Input: part model. Units: mm. Frame: model coordinates. A direction names the side the tool comes from. Coordinates: 2 decimals unless noted, no trailing zeros. Order: outer loops, then holes, each group sorted by start corner. A loop starts at its lowest first (then second) coordinate and runs counter-clockwise, first axis right, second up. Notation, with made-up numbers: (-14, 71.5) -> (4, 71.5) arc R14 cw to (4, 85.5) -> close; hole circle Ø7 at (53.5, 77). An arc over 180 degrees is marked (long way). Use one line per item in the form item = value. Start each with the question number.
1) Section query A-A on x = 24. Output: boundary loops of the cut face in (y, z).
2) Pin query (flat end, axial travel): pin 1 (1 mm diameter, centred on y = -1, z = -38, fed in from -X); pin 2 (10 mm diameter, centred on x = -24, z = -41, fed in from -Y); pin 3 (2 mm diameter, centred on x = 9.5, z = -51.5, fed in from +Y). Return the tip coordinate at first contact, or that it passes through.
3) Draft query along X for faces 1 (the cylindrical face through (43.998, 0.325, -57.664)), 2 (the cylindrical face through (-5.9, -44.934, -29.58)), 3 (the cylindrical face through (0.9, 44, -55)). Return one class per face: pulls with the +X half, pulls with the -X half, needs draft (parallel to the pull), parting line crosses it, or undercut.
4) Section query D-D on y = -6.5. Output: boundary loops of the cut face in (x, z).
5) Section query B-B on y = 12. Output: boundary loops of the cut face in (x, z), then the cut area to 3 significant figures.
6) Section query C-C on z = -35.2. Output: boundary loops of the cut face in (x, y) (3 decimals).
7) Ray query, line 1 along Z through (x, y) = (0, 43.95); line 2 along Z through (x, y) = (0, -43.8); line 3 along Y through (x, z) = (0, -28.5) (3 decimals). Return the intervals inside material, ascending.
8) Access query for faces 4 (the flat face through (44, 1.5, -9)), 5 (the cylindrical face through (40.7, -12.8, -29.6)), 6 (the flat face through (1.5, 44, -9)). Directions: +Z, -Z, +X, -X, +Y, -Y. A direction counts if a zero-diameter tool reaches every point of the face in a straight line with its end or side. Return the directions, or none.
from build123d import *

# Parameters (mm, degrees)
SKETCH_R             = 45.32
SKETCH_R_2           = 42.665
PAD_DEPTH            = 60
SKETCH002_R          = 1.5
SKETCH002_R_2        = 10
POCKET_DEPTH         = 8
SKETCH003_R          = 1.5
POCKET001_DEPTH      = 8
SKETCH004_R          = 1.5
POCKET002_DEPTH      = 5
BODY_PLACEMENT_ANGLE = 180


with BuildPart() as part:
    # Sketch → Pad (new body)
    with BuildSketch(Plane.XY):
        Circle(SKETCH_R)
        Circle(SKETCH_R_2, mode=Mode.SUBTRACT)
    extrude(amount=PAD_DEPTH)

    # Sketch002 (on DatumPlane) → Pocket (cut)
    with BuildSketch(Plane(origin=(45.32, 0, 60), x_dir=(0, 1, 0), z_dir=(-1, 0, 0))):
        with Locations((0, 3.8)):
            Circle(SKETCH002_R)
        with Locations((0, 18)):
            Circle(SKETCH002_R_2)
        with BuildLine():
            Line((0, 47.6), (0.0005, 47.6))
            ThreePointArc((0.0005, 47.6), (1.060807, 48.039193), (1.5, 49.0995))
            Line((1.5, 49.0995), (1.5, 52.1005))
            ThreePointArc((1.5, 52.1005), (1.060807, 53.160807), (0.0005, 53.6))
            Line((0.0005, 53.6), (0, 53.6))
            ThreePointArc((0, 53.6), (-1.06066, 53.16066), (-1.5, 52.1))
            Line((-1.5, 52.1), (-1.5, 49.1))
            ThreePointArc((-1.5, 49.1), (-1.06066, 48.03934), (0, 47.6))
        make_face()
    extrude(amount=POCKET_DEPTH, mode=Mode.SUBTRACT)

    # Sketch003 (on DatumPlane) → Pocket001 (cut)
    with BuildSketch(Plane(origin=(0, 45.32, 60), x_dir=(0, 0, -1), z_dir=(0, 1, 0))):
        with Locations((3.8, 0)):
            Circle(SKETCH003_R)
        with Locations((24.8, 0)):
            Circle(SKETCH003_R)
    extrude(amount=-POCKET001_DEPTH, mode=Mode.SUBTRACT)

    # Sketch004 (on DatumPlane) → Pocket002 (cut)
    with BuildSketch(Plane(origin=(0, -45.32, 60), x_dir=(0, 0, 1), z_dir=(0, -1, 0))):
        with Locations((-3.8, 0)):
            Circle(SKETCH004_R)
        with Locations((-24.8, 0)):
            Circle(SKETCH004_R)
        with BuildLine():
            Line((-52.1, -1.5), (-49.095, -1.5))
            ThreePointArc((-49.095, -1.5), (-48.037875, -1.062125), (-47.6, -0.005))
            Line((-47.6, -0.005), (-47.6, 0))
            ThreePointArc((-47.6, 0), (-48.03934, 1.06066), (-49.1, 1.5))
            Line((-49.1, 1.5), (-52.105, 1.5))
            ThreePointArc((-52.105, 1.5), (-53.162125, 1.062125), (-53.6, 0.005))
            Line((-53.6, 0.005), (-53.6, 0))
            ThreePointArc((-53.6, 0), (-53.16066, -1.06066), (-52.1, -1.5))
        make_face()
    extrude(amount=-POCKET002_DEPTH, mode=Mode.SUBTRACT)


with BuildPart() as part_1:
    # Body placement: moved
    add(part.part.rotate(Axis((0, 0, 0), (1, 0, 0)), BODY_PLACEMENT_ANGLE))


solid = part_1.part
Answers below:
q1.outline = (-38.44, -60) -> (-35.27, -60) -> (-35.27, 0) -> (-38.44, 0) -> close; (35.27, -60) -> (38.44, -60) -> (38.44, 0) -> (35.27, 0) -> close
q2.pin_1 = -45.32
q2.pin_2 = -41.14
q2.pin_3 = 44.52
q3.face_1 = needs draft
q3.face_2 = parting line crosses it
q3.face_3 = undercut
q4.outline = (-44.85, -60) -> (-42.17, -60) -> (-42.17, 0) -> (-44.85, 0) -> close; (42.17, -60) -> (44.85, -60) -> (44.85, -49.6) -> (42.17, -49.6) -> close; (42.17, -34.4) -> (44.85, -34.4) -> (44.85, 0) -> (42.17, 0) -> close
q5.outline = (-43.7, -60) -> (-40.94, -60) -> (-40.94, 0) -> (-43.7, 0) -> close; (40.94, -60) -> (43.7, -60) -> (43.7, 0) -> (40.94, 0) -> close
q5.area = 331 mm^2
q6.outline = (-1.5, -45.295) -> (-1.5, -42.639) arc R42.665 cw to (-1.5, 42.639) -> (-1.5, 45.295) arc R45.32 ccw to start; (1.5, -45.295) arc R45.32 ccw to (44.723, -7.332) -> (42.03, -7.332) arc R42.665 cw to (1.5, -42.639) -> close; (1.5, 42.639) arc R42.665 cw to (42.03, 7.332) -> (44.723, 7.332) arc R45.32 ccw to (1.5, 45.295) -> close
q7.line_1 = -60 to -57.7, -54.7 to -36.7, -33.7 to -12.4, -6.4 to 0
q7.line_2 = -60 to -57.7, -54.7 to -36.7, -33.7 to 0
q7.line_3 = -45.32 to -42.665, 42.665 to 45.32
q8.face_4 = +X
q8.face_5 = +Z, -Z
q8.face_6 = +Y
